For this review, take the finished solid that the model builds, in its own axes (mm). A direction names the side the tool comes from. Give positions to 0.01 mm unless a question says otherwise; leave off trailing zeros. Loops run counter-clockwise (first coordinate to the right, second up) from the corner with the lowest first, then second, coordinate; pieces in that order, holes last. Notation, with made-up numbers: (6.5, 35) - (52.5, 35) arc R37 cw to (52.5, 73) - close; hole circle Ø5 at (32.5, -39.75). An arc over 180 degrees is marked (long way). Answer as CSV lines item,"result".
from build123d import *

# Parameters (mm, degrees)
BOSS_EXTRUDE1_DEPTH = 19.05
FILLET3_R           = 2.54


with BuildPart() as part:
    # Sketch1 → Boss-Extrude1 (new body)
    with BuildSketch(Plane(origin=(0, 0, 0), x_dir=(0, 0, -1), z_dir=(1, 0, 0))):
        Polygon((0, -27.94), (0, 0), (9.5504, 0), (9.5504, -27.94), (14.6304, -27.94), (14.6304, 12.7), (-12.7, 12.7), (-12.7, -27.94), align=None)
    extrude(amount=BOSS_EXTRUDE1_DEPTH)

    # Fillet3
    fillet3_edges = [part.edges().sort_by_distance(p)[0] for p in [
        (9.525, -27.94, 12.7),
        (9.525, 12.7, 12.7),
        (9.525, 12.7, -14.6304),
        (9.525, -27.94, -14.6304),
        (9.525, -27.94, -9.5504),
        (9.525, -27.94, 0),
    ]]
    fillet(fillet3_edges, radius=FILLET3_R - 0.0001)  # a hair under: the kernel refuses the full size


solid = part.part
1) Consider section D-D on z = 0.75. Write out the cut boundary in (x, y), and give its area (3 significant figures).
From the geometry:
outline,"(0, -27.2) - (19.05, -27.2) - (19.05, 12.7) - (0, 12.7) - close"
area,"760 mm^2"
2) Consider section A-A on y = -3. Write out the cut boundary in (x, z).
From the geometry:
outline,"(0, -14.63) - (19.05, -14.63) - (19.05, -9.55) - (0, -9.55) - close; (0, 0) - (19.05, 0) - (19.05, 12.7) - (0, 12.7) - close"
3) Consider section C-C on z = -5.25. Write out the cut boundary in (x, y), and give its area (3 significant figures).
From the geometry:
outline,"(0, 0) - (19.05, 0) - (19.05, 12.7) - (0, 12.7) - close"
area,"242 mm^2"
4) Machinability: for faces 5 (the flat face through (9, -13, -9.55)), 6 (the cylindrical face through (9.658, 11.936, -13.906)), which of the approach directions +Z, -Z, +X, -X, +Y, -Y give a long, thin tool a straight path to every point of the face, cutting with its end or side? Answer none if there is none.
From the geometry:
face 5,"+X, -X, -Y"
face 6,"-Z, +X, -X, +Y"
5) Wall thickness on line 1 (Z direction, x = 18, y = -13); line 2 (Y direction, x = 17.75, z = -6); line 3 (Z direction, x = 9.5, y = 10.5): over which ranges is each line inside the solid? List them lowest first. Write a range as from..to.
From the geometry:
line 1,"z = -14.63..-9.55, 0..12.7"
line 2,"y = 0..12.7"
line 3,"z = -14.61..12.68"
6) Insertion check: P1, Ø5, axis at x = 7.5, z = -4.5, coming from the -Y side. The pin has a flat end and moves straight along its axis. Give the tip position at first contact, or say it passes through.
From the geometry:
P1,"stops at y = 0"
7) Draft analysis for pull direction Z (two halves, no side actions). For faces 1 (the flat face through (9, 0, -5)), 2 (the cylindrical face through (9.658, 11.976, 11.936)), 3 (the flat face through (0, -7, 2)), 4 (the flat face through (9, -13, 0)), state which applies: pulls with the +Z half, pulls with the -Z half, needs draft (parallel to the pull), parting line crosses it, or undercut.
From the geometry:
face 1,"undercut"
face 2,"pulls with the +Z half"
face 3,"needs draft"
face 4,"undercut"
